CAD build for the part. Positions are in the model's coordinates, mm. Face numbers are marked on the shaded views. A direction names the side the tool comes from. Round coordinates to 2 decimals unless told otherwise and drop trailing zeros. Write each loop counter-clockwise with the first axis right and the second up, starting at its lowest first coordinate (ties: lowest second). Pieces come first, ordered by that corner, then holes. Notation, with made-up numbers: (-23, -4.5) - (-2, -4.5) arc R28 ccw to (-2, 23.5) - close; hole circle Ø5 at (77, -10.75). An arc over 180 degrees is marked (long way). Use one line per item in the form item = value. Start each with the question number.
Item 1: Band-saw the part on A-A, the plane z = 1.5. List the corners of the cut face in (x, y), and give its area (3 significant figures).
Item 2: Tool access for the marked faces 1 and 2: list every direction of +Z, -Z, +X, -X, +Y, -Y with a clear straight run to the whole face (end or side of a thin tool).
Item 3: Drill centre lines: L1, parallel to Y at x = 0, z = 10.5; L2, parallel to Z at x = 6, y = 14; L3, parallel to Y at x = -1.5, z = 3. Where is each one in solid material? Low to high.
Item 4: Band-saw the part on B-B, the plane y = -16. List the corners of the cut face in (x, z).
Item 5: Pin check, flat tips, straight feed: pin 1 (10 mm diameter, centred on y = 1.5, z = 14.5, fed in from +X); pin 2 (6.5 mm diameter, centred on x = 0, y = 0, fed in from +Z); pin 3 (10 mm diameter, centred on y = 11.5, z = 8.5, fed in from -X); pin 4 (1 mm diameter, centred on x = -8, z = 14.5, fed in from +Y). Stop position of each tip, or through.
Item 6: Pull direction X, two halves, no side cores. Call the marked faces 3, 4 and 5: +X half, -X half, draft (parallel to the pull), parting line (faces both ways), or undercut.
Item 7: Band-saw the part on D-D, the plane y = -5. List the corners of the cut face in (x, z).
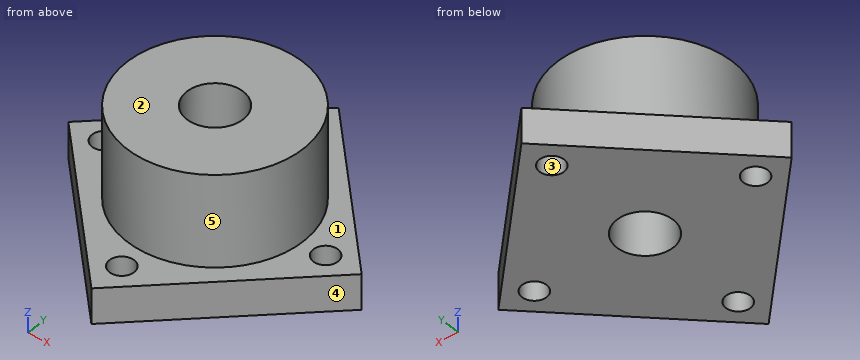
from build123d import *

# Parameters (mm, degrees)
SKETCH_1_R          = 4
EXTRUDE_1_DEPTH     = 5
SKETCH_2_R          = 1.75
CUT_EXTRUDE_1_DEPTH = 5
SKETCH_3_R          = 12.5
SKETCH_3_R_2        = 4
EXTRUDE_2_DEPTH     = 13


with BuildPart() as part:
    # 草图1 → 凸台-拉伸1 (new body)
    with BuildSketch(Plane.XY):
        Polygon((0, 21.213203436), (-21.213203436, 0), (0, -21.213203436), (21.213203436, 0), align=None)
        Circle(SKETCH_1_R, mode=Mode.SUBTRACT)
    extrude(amount=EXTRUDE_1_DEPTH)

    # 草图2 → 切除-拉伸1 (cut)
    with BuildSketch(Plane.XY.offset(5)):
        with Locations((16, 0)):
            Circle(SKETCH_2_R)
        with Locations((0, -16)):
            Circle(SKETCH_2_R)
        with Locations((-16, 0)):
            Circle(SKETCH_2_R)
        with Locations((0, 16)):
            Circle(SKETCH_2_R)
    extrude(amount=-CUT_EXTRUDE_1_DEPTH, mode=Mode.SUBTRACT)

    # 草图3 → 凸台-拉伸2 (add)
    with BuildSketch(Plane.XY.offset(5)):
        with Locations(Location((0, 0, 0), (0, 0, 180))):
            Circle(SKETCH_3_R)
        Circle(SKETCH_3_R_2, mode=Mode.SUBTRACT)
    extrude(amount=EXTRUDE_2_DEPTH)


solid = part.part
Determined:
q1.outline = (-21.21, 0) - (0, -21.21) - (21.21, 0) - (0, 21.21) - close; hole circle Ø3.5 at (-16, 0); hole circle Ø8 at (0, 0); hole circle Ø3.5 at (0, -16); hole circle Ø3.5 at (0, 16); hole circle Ø3.5 at (16, 0)
q1.area = 811 mm²
q2.face_1 = +Z
q2.face_2 = +Z, +X, -X, +Y, -Y
q3.L1 = -12.5 to -4, 4 to 12.5
q3.L2 = 0 to 5
q3.L3 = -19.71 to -16.9, -15.1 to -3.71, 3.71 to 15.1, 16.9 to 19.71
q4.outline = (-5.21, 0) - (-1.75, 0) - (-1.75, 5) - (-5.21, 5) - close; (1.75, 0) - (5.21, 0) - (5.21, 5) - (1.75, 5) - close
q5.pin_1 = 12.5
q5.pin_2 = through
q5.pin_3 = -13.28
q5.pin_4 = 10
q6.face_3 = undercut
q6.face_4 = +X half
q6.face_5 = parting line
q7.outline = (-16.21, 0) - (16.21, 0) - (16.21, 5) - (11.46, 5) - (11.46, 18) - (-11.46, 18) - (-11.46, 5) - (-16.21, 5) - close
